from build123d import *

# Parameters (mm, degrees)
SKETCH1_R              = 18.5
BOSS_EXTRUDE1_DEPTH    = 6
SKETCH2_R              = 18.5
SKETCH2_R_2            = 17.5
BOSS_EXTRUDE2_DEPTH    = 1
M14X1_5_TAPPED_HOLE1_D = 12.5
SKETCH5_R              = 2.25
CUT_EXTRUDE1_DEPTH     = 4


with BuildPart() as part:
    # Sketch1 → Boss-Extrude1 (new body)
    with BuildSketch(Plane(origin=(0, 0, 0), x_dir=(1, 0, 0), z_dir=(0, 1, 0))):
        Circle(SKETCH1_R)
    extrude(amount=BOSS_EXTRUDE1_DEPTH)

    # Sketch2 → Boss-Extrude2 (add)
    with BuildSketch(Plane(origin=(0, 6, 0), x_dir=(1, 0, 0), z_dir=(0, 1, 0))):
        Circle(SKETCH2_R)
        Circle(SKETCH2_R_2, mode=Mode.SUBTRACT)
    extrude(amount=BOSS_EXTRUDE2_DEPTH)

    # M14x1.5 Tapped Hole1 (through all)
    with Locations(Plane(origin=(0, 6, 0), x_dir=(1, 0, 0), z_dir=(0, 1, 0))):
        with Locations((0, 0)):
            Hole(M14X1_5_TAPPED_HOLE1_D / 2)

    # Sketch5 → Cut-Extrude1 (cut)
    with BuildSketch(Plane.XZ):
        with Locations((-10.606601718, 10.606601718)):
            Circle(SKETCH5_R)
        with Locations((10.606601718, 10.606601718)):
            Circle(SKETCH5_R)
        with Locations((10.606601718, -10.606601718)):
            Circle(SKETCH5_R)
        with Locations((-10.606601718, -10.606601718)):
            Circle(SKETCH5_R)
    extrude(amount=-CUT_EXTRUDE1_DEPTH, mode=Mode.SUBTRACT)


solid = part.part
Design review of the part built by this model. Coordinates are the model's own, in mm. A direction names the side the tool comes from. Coordinates: 2 decimals unless noted, no trailing zeros. Loops run counter-clockwise (first coordinate to the right, second up) from the corner with the lowest first, then second, coordinate; pieces in that order, holes last. Notation, with made-up numbers: (69.5, 80) - (109.5, 80) arc R25 ccw to (109.5, 115) - close; hole circle Ø6 at (29, -4). An arc over 180 degrees is marked (long way). Use CSV: the item, a comma, the result in double quotes. Start each with the question number.
1. Mouldability with a two-part tool opening along X and no side actions: class faces 1 (the cylindrical face through (8.95, 1.97, 12.13)), 2 (the flat face through (8, 0, 0)), 3 (the cylindrical face through (-13.887, 6.493, 10.648)), 4 (the cylindrical face through (-4.01, 3.45, 18.06)) as released by +X, released by -X, zero draft, split by the parting line, or undercut.
2. Clearance check with flat-ended pins moving along their axes: pin 1 (17.5 mm diameter, centred on x = 0, z = -5.5, fed in from +Y); pin 2 (1.5 mm diameter, centred on x = -3.5, y = 2, fed in from +Z); pin 3 (2 mm diameter, centred on x = 2.5, y = 4.5, fed in from -Z). State where each tip first meets the part, or that it passes through.
3. Add section A-A on z = 0. Give the boundary of the cut face in (x, y).
4. For faces 5 (the cylindrical face through (-9.397, 1.972, 12.504)), 6 (the flat face through (-11, 7, 14)), 7 (the flat face through (0, 6, 8)), list the 3-axis set-ups (+Z, -Z, +X, -X, +Y, -Y) from which the entire face can be reached by the end or side of a thin tool; tool diameter is ignored.
5. To check wall thickness, follow probe 1 along Z at (x, y) = (11, 1.5); probe 2 along X at (y, z) = (1.75, -9.5). State the ranges of each line that lie inside material, in increasing order.
6. Add section D-D on y = 1.25. Give the boundary of the cut face in (x, z), plus the area to 3 significant figures.
7. Add section C-C on y = 5.25. Give the boundary of the cut face in (x, z), plus the area to 3 significant figures.
8. Add section B-B on x = 0. Give the boundary of the cut face in (y, z).
Resolved:
1,face 1,"undercut"
1,face 2,"zero draft"
1,face 3,"undercut"
1,face 4,"split by the parting line"
2,pin 1,"y = 6"
2,pin 2,"z = 18.29"
2,pin 3,"z = -18.44"
3,outline,"(-18.5, 0) - (-6.25, 0) - (-6.25, 6) - (-17.5, 6) - (-17.5, 7) - (-18.5, 7) - close; (6.25, 0) - (18.5, 0) - (18.5, 7) - (17.5, 7) - (17.5, 6) - (6.25, 6) - close"
4,face 5,"-Y"
4,face 6,"+Z, -Z, +X, -X, +Y"
4,face 7,"+Y"
5,probe 1,"-14.87 to -12.82, -8.39 to 8.39, 12.82 to 14.87"
5,probe 2,"-15.87 to -12.57, -8.65 to 8.65, 12.57 to 15.87"
6,outline,"circle Ø37 at (0, 0); hole circle Ø4.5 at (-10.61, -10.61); hole circle Ø4.5 at (-10.61, 10.61); hole circle Ø12.5 at (0, 0); hole circle Ø4.5 at (10.61, -10.61); hole circle Ø4.5 at (10.61, 10.61)"
6,area,"889 mm2"
7,outline,"circle Ø37 at (0, 0); hole circle Ø12.5 at (0, 0)"
7,area,"952 mm2"
8,outline,"(0, -18.5) - (7, -18.5) - (7, -17.5) - (6, -17.5) - (6, -6.25) - (0, -6.25) - close; (0, 6.25) - (6, 6.25) - (6, 17.5) - (7, 17.5) - (7, 18.5) - (0, 18.5) - close"
